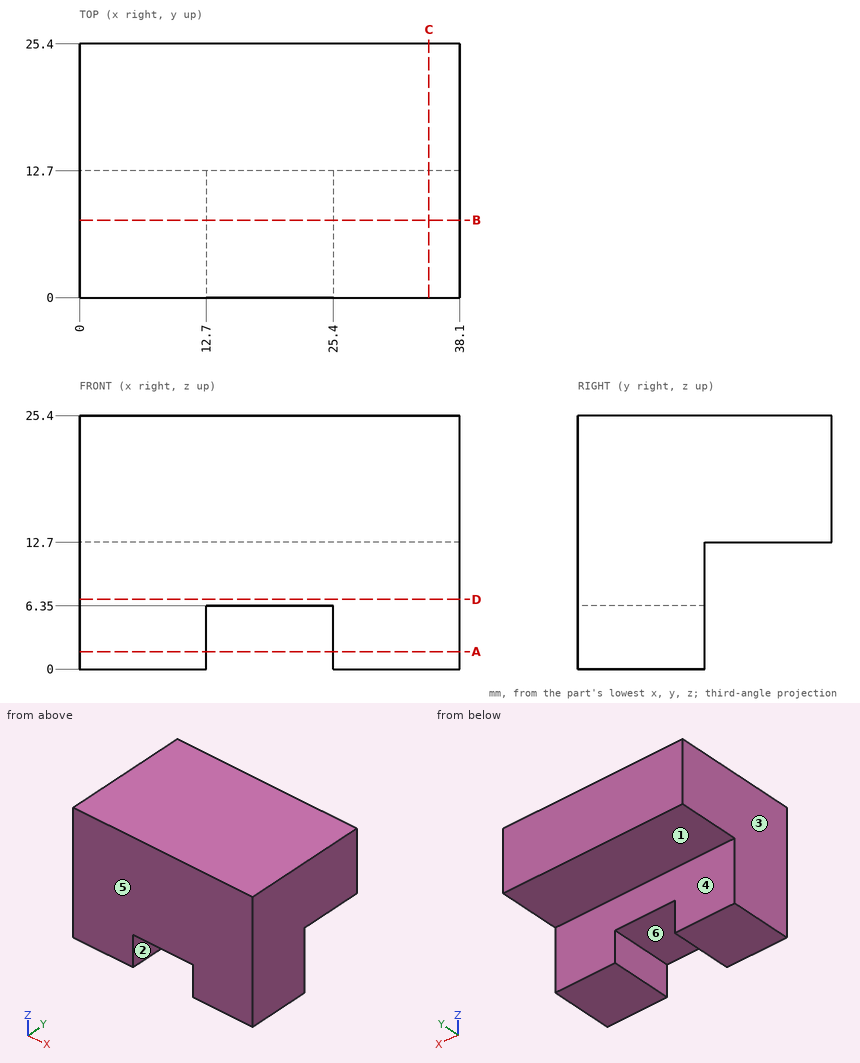
Verification items for this drawing (mm, ordinates from the low corner). A direction names the side the tool comes from. Round coordinates to 2 decimals unless told otherwise and drop trailing zeros. Loops run counter-clockwise (first coordinate to the right, second up) from the corner with the lowest first, then second, coordinate; pieces in that order, holes last. Notation, with made-up numbers: (-7, -1.75) -> (17, -1.75) arc R25 ccw to (17, 25.25) -> close; hole circle Ø9 at (69, 58.5). An arc over 180 degrees is marked (long way). Answer in a Markdown table with one row per item.
Q1. Sectioned sample at B-B on y = 7.75. Enter the section's corners in (x, z).
Data:
| item | result |
|---|---|
| outline | (0, 0) -> (12.7, 0) -> (12.7, 6.35) -> (25.4, 6.35) -> (25.4, 0) -> (38.1, 0) -> (38.1, 25.4) -> (0, 25.4) -> close |
Q2. Set-up check for the marked faces 4, 5 and 6: record each of +Z, -Z, +X, -X, +Y, -Y from which the full face is reachable in a straight line by a thin tool's end or side.
Data:
| item | result |
|---|---|
| face 4 | -Z, +X, -X, +Y |
| face 5 | +Z, -Z, +X, -X, -Y |
| face 6 | -Z, +Y, -Y |
Q3. Sectioned sample at C-C on x = 35. Enter the section's corners in (y, z), then the cut area to 3 significant figures.
Data:
| item | result |
|---|---|
| outline | (0, 0) -> (12.7, 0) -> (12.7, 12.7) -> (25.4, 12.7) -> (25.4, 25.4) -> (0, 25.4) -> close |
| area | 484 mm^2 |
Q4. Thickness scan on L1, parallel to X at y = 2.75, z = 2; L2, parallel to Z at x = 4, y = 22.5; L3, parallel to Y at x = 32.5, z = 8.75. Record the ranges inside material, lowest first.
Data:
| item | result |
|---|---|
| L1 | x = 0 to 12.7, 25.4 to 38.1 |
| L2 | z = 12.7 to 25.4 |
| L3 | y = 0 to 12.7 |
Q5. Sectioned sample at D-D on z = 7. Enter the section's corners in (x, y).
Data:
| item | result |
|---|---|
| outline | (0, 0) -> (38.1, 0) -> (38.1, 12.7) -> (0, 12.7) -> close |
Q6. Sectioned sample at A-A on z = 1.75. Enter the section's corners in (x, y), then the cut area to 3 significant figures.
Data:
| item | result |
|---|---|
| outline | (0, 0) -> (12.7, 0) -> (12.7, 12.7) -> (0, 12.7) -> close; (25.4, 0) -> (38.1, 0) -> (38.1, 12.7) -> (25.4, 12.7) -> close |
| area | 323 mm^2 |
Q7. Go/stop test with flat-tipped pins: P1, Ø4, axis at x = 22, y = 17.5, coming from the -Z side; P2, Ø14, axis at x = 14, z = 5, coming from the +Y side. Record where each tip stops, or that it passes through.
Data:
| item | result |
|---|---|
| P1 | stops at z = 12.7 |
| P2 | stops at y = 12.7 |
Q8. Release check for a two-part mould opening along X. For the marked faces 1, 2 and 3 record: released by +X, released by -X, zero draft, split by the parting line, or undercut.
Data:
| item | result |
|---|---|
| face 1 | zero draft |
| face 2 | undercut |
| face 3 | released by -X |
